Verification items for the finished model (mm, model axes). A direction names the side the tool comes from. Give positions to 0.01 mm unless a question says otherwise; leave off trailing zeros. Loops run counter-clockwise (first coordinate to the right, second up) from the corner with the lowest first, then second, coordinate; pieces in that order, holes last. Notation, with made-up numbers: (13.5, 4.5) - (35.5, 4.5) arc R22 ccw to (35.5, 16.5) - close; hole circle Ø11 at (24.25, 63). An arc over 180 degrees is marked (long way). Answer in a Markdown table with one row per item.
```python
from build123d import *

# Parameters (mm, degrees)
SKETCH7_W               = 25
SKETCH7_H               = 10
SKETCH7_R               = 1.6
BOSS_EXTRUDE3_DEPTH     = 3
SKETCH8_W               = 25
SKETCH8_H               = 3
BOSS_EXTRUDE4_DEPTH     = 24
CUT_EXTRUDE5_DEPTH      = 5
SKETCH10_OUTSIDE_W      = 34.626
SKETCH10_OUTSIDE_H      = 36.626
CUT_EXTRUDE6_DEPTH      = 5
SKETCH11_W              = 10
SKETCH11_H              = 8
BOSS_EXTRUDE5_DEPTH     = 1
CHAMFER1_SIZE           = 2
CHAMFER1_SIZE2          = 5.494954839
CHAMFER1_PART_2_SIZE    = 2
CHAMFER1_PART_2_SIZE2   = 5.494954839
CUT_EXTRUDE7_DEPTH      = 1.3
SKETCH14_W              = 3.2
SKETCH14_H              = 3.813108433
CUT_EXTRUDE9_DEPTH      = 2.3
CUT_EXTRUDE9_DEPTH_BACK = 10.7
FILLET3_R               = 10


with BuildPart() as part:
    # Sketch7 → Boss-Extrude3 (new body)
    with BuildSketch(Plane(origin=(0, 0, 0), x_dir=(1, 0, 0), z_dir=(0, 1, 0))):
        Rectangle(SKETCH7_W, SKETCH7_H)
        with Locations(Location((-10, 2.276747262, 0), (0, 0, 270))):  # turned: the seam where the file's is
            Circle(SKETCH7_R, mode=Mode.SUBTRACT)
        with Locations(Location((10, 2.276747262, 0), (0, 0, 270))):  # turned: the seam where the file's is
            Circle(SKETCH7_R, mode=Mode.SUBTRACT)
    extrude(amount=BOSS_EXTRUDE3_DEPTH)

    # Sketch8 → Boss-Extrude4 (add)
    with BuildSketch(Plane(origin=(0, 3, 0), x_dir=(1, 0, 0), z_dir=(0, 1, 0))):
        with Locations((0, -3.5)):
            Rectangle(SKETCH8_W, SKETCH8_H)
    extrude(amount=BOSS_EXTRUDE4_DEPTH)

    # Sketch9 → Cut-Extrude5 (cut)
    with BuildSketch(Plane.XY.offset(5)):
        Polygon((8, 8), (8, 0), (-8, 0), (-8, 8), (-3, 8), (-3, 18), (3, 18), (3, 8), align=None)
    extrude(amount=-CUT_EXTRUDE5_DEPTH, mode=Mode.SUBTRACT)

    # Sketch10 outside → Cut-Extrude6 (cut)
    with BuildSketch(Plane.XY.offset(5)):
        with Locations((0, 13.5)):
            Rectangle(SKETCH10_OUTSIDE_W, SKETCH10_OUTSIDE_H)
        Polygon((-5, 27), (-5, 12), (-12.5, 8), (-12.5, 0), (12.5, 0), (12.5, 8), (5, 12), (5, 27), align=None, mode=Mode.SUBTRACT)
    extrude(amount=-CUT_EXTRUDE6_DEPTH, mode=Mode.SUBTRACT)

    # Sketch11 → Boss-Extrude5 (add)
    with BuildSketch(Plane.XY.offset(5)):
        with Locations((0, 23)):
            Rectangle(SKETCH11_W, SKETCH11_H)
    extrude(amount=BOSS_EXTRUDE5_DEPTH)

    # Chamfer1
    chamfer1_edges = [part.edges().sort_by_distance(p)[0] for p in [
        (-3, 8, 3.5),
    ]]
    chamfer1_side = [part.faces().sort_by_distance(p)[0] for p in [
        (-5.5, 8, 3.5),
    ]]
    chamfer(chamfer1_edges, length=CHAMFER1_SIZE, length2=CHAMFER1_SIZE2, reference=chamfer1_side[0])

    # Chamfer1 part 2
    chamfer1_part_2_edges = [part.edges().sort_by_distance(p)[0] for p in [
        (3, 8, 3.5),
    ]]
    chamfer1_part_2_side = [part.faces().sort_by_distance(p)[0] for p in [
        (5.5, 8, 3.5),
    ]]
    chamfer(chamfer1_part_2_edges, length=CHAMFER1_PART_2_SIZE, length2=CHAMFER1_PART_2_SIZE2, reference=chamfer1_part_2_side[0])

    # Sketch12 → Cut-Extrude7 (cut)
    with BuildSketch(Plane.XY.offset(6)):
        Polygon((-2.2, 20.45), (-1.6, 20.45), (-1.6, 19), (1.6, 19), (1.6, 20.45), (2.2, 20.45), (2.2, 23.55), (-2.2, 23.55), align=None)
    extrude(amount=-CUT_EXTRUDE7_DEPTH, mode=Mode.SUBTRACT)

    # Sketch14 → Cut-Extrude9 (cut, two sides)
    with BuildSketch(Plane.XY.offset(4.7)) as cut_extrude9_sk:
        with Locations((0, 18.543445784)):
            Rectangle(SKETCH14_W, SKETCH14_H)
    extrude(amount=CUT_EXTRUDE9_DEPTH, mode=Mode.SUBTRACT)
    extrude(cut_extrude9_sk.sketch, amount=-CUT_EXTRUDE9_DEPTH_BACK, mode=Mode.SUBTRACT)

    # Fillet3
    fillet3_edges = [part.edges().sort_by_distance(p)[0] for p in [
        (-5, 12, 3.5),
        (5, 12, 3.5),
    ]]
    fillet(fillet3_edges, radius=FILLET3_R)


solid = part.part
```
Q1. Draft check along X on faces 4 (the face through (-11.382, 8.596, 3.521)), 5 (the face through (-2, 18, 4)), 6 (the face through (0, 3, -2)). Enter one of: +X half, -X half, draft (parallel to the pull), parting line (faces both ways), or undercut.
Completed:
| item | result |
|---|---|
| face 4 | -X half |
| face 5 | undercut |
| face 6 | draft |
Q2. Sectioned sample at C-C (z = -1.25). Record the cut outline in (x, y), and give its area (3 significant figures).
Completed:
| item | result |
|---|---|
| outline | (-12.5, 0) - (-11.23, 0) - (-11.23, 3) - (-12.5, 3) - close; (-8.77, 0) - (8.77, 0) - (8.77, 3) - (-8.77, 3) - close; (11.23, 0) - (12.5, 0) - (12.5, 3) - (11.23, 3) - close |
| area | 60.3 mm^2 |
Q3. Tool access check on faces 1 (the face through (8.2, 7.3, 5)), 2 (the face through (0, 23.55, 5)), 3 (the face through (8, 3, 3)). Record the directions out of +Z, -Z, +X, -X, +Y, -Y that give a thin tool (end or side, any length) a straight path to the whole face; none if there is none.
Completed:
| item | result |
|---|---|
| face 1 | +Z, +X, -X, -Y |
| face 2 | +Z |
| face 3 | +Z, -Y |
Q4. Sectioned sample at B-B (x = -0.25). Record the cut outline in (y, z).
Completed:
| item | result |
|---|---|
| outline | (0, -5) - (3, -5) - (3, 0) - (0, 0) - close; (20.45, 2) - (27, 2) - (27, 6) - (23.55, 6) - (23.55, 4.7) - (20.45, 4.7) - close |
Q5. Thickness scan on line 1 (X direction, y = 6.5, z = 4); line 2 (X direction, y = 20, z = 5.25); line 3 (Z direction, x = -4, y = 12). Record the ranges inside material, lowest first.
Completed:
| item | result |
|---|---|
| line 1 | -12.5 to -8, 8 to 12.5 |
| line 2 | -5 to -1.6, 1.6 to 5 |
| line 3 | 2 to 5 |
Q6. Sectioned sample at D-D (y = 2.25). Record the cut outline in (x, z), and give its area (3 significant figures).
Completed:
| item | result |
|---|---|
| outline | (-12.5, -5) - (12.5, -5) - (12.5, 5) - (8, 5) - (8, 0) - (-8, 0) - (-8, 5) - (-12.5, 5) - close; hole circle Ø3.2 at (-10, -2.28); hole circle Ø3.2 at (10, -2.28) |
| area | 154 mm^2 |
Q7. Sectioned sample at A-A (y = 6.25). Record the cut outline in (x, z), and give its area (3 significant figures).
Completed:
| item | result |
|---|---|
| outline | (-12.5, 2) - (-8, 2) - (-8, 5) - (-12.5, 5) - close; (8, 2) - (12.5, 2) - (12.5, 5) - (8, 5) - close |
| area | 27.0 mm^2 |
Q8. Go/stop test with flat-tipped pins: P1, Ø5, axis at x = 1, y = 7.5, coming from the +Z side; P2, Ø0.9, axis at x = -2, y = 2, coming from the +Z side; P3, Ø1, axis at y = 17.5, z = 3.5, coming from the -X side; P4, Ø2, axis at y = 21, z = 3.5, coming from the -X side. Record where each tip stops, or that it passes through.
Completed:
| item | result |
|---|---|
| P1 | through |
| P2 | z = 0 |
| P3 | x = -5.05 |
| P4 | x = -5 |
